Here's how the part is built. I have some questions about the finished solid (model axes, mm). Face numbers are marked on the shaded views. A direction names the side the tool comes from. Give positions to 0.01 mm unless a question says otherwise; leave off trailing zeros. Order: outer loops, then holes, each group sorted by start corner. A loop starts at its lowest first (then second) coordinate and runs counter-clockwise, first axis right, second up. Notation, with made-up numbers: M 69.25,-31.5 L 103.25,-31.5 A12 ccw 103.25,-23.5 Z; hole C -14,45 d4. An arc over 180 degrees is marked long. Use one line per item in the form item = value.
from build123d import *

# Parameters (mm, degrees)
F0_W     = 200
F0_H     = 200
F0_W_2   = 800
F0_H_2   = 800
F1_DEPTH = 200
F2_DEPTH = 300
F3_DEPTH = 200.001
F4_W     = 1200
F4_H     = 1200
F4_W_2   = 800
F4_H_2   = 800
F5_DEPTH = 200


with BuildPart() as f1:
    # F0 (on Top) → F1 (new body)
    with BuildSketch(Plane.XY):
        with Locations((-500, 500)):
            Rectangle(F0_W, F0_H)
        with Locations((0, 500)):
            Rectangle(F0_W_2, F0_H)
        with Locations((500, 500)):
            Rectangle(F0_W, F0_H)
        with Locations((500, 0)):
            Rectangle(F0_W, F0_H_2)
        Rectangle(F0_W_2, F0_H_2)
        with Locations((-500, 0)):
            Rectangle(F0_W, F0_H_2)
        with Locations((-500, -500)):
            Rectangle(F0_W, F0_H)
        with Locations((0, -500)):
            Rectangle(F0_W_2, F0_H)
        with Locations((500, -500)):
            Rectangle(F0_W, F0_H)
    extrude(amount=-F1_DEPTH)

    # F0 (on Top) → F2 (join)
    with BuildSketch(Plane.XY):
        with Locations((-500, -500)):
            Rectangle(F0_W, F0_H)
        with Locations((500, -500)):
            Rectangle(F0_W, F0_H)
        with Locations((500, 500)):
            Rectangle(F0_W, F0_H)
        with Locations((-500, 500)):
            Rectangle(F0_W, F0_H)
    extrude(amount=F2_DEPTH)

    # F0 (on Top) → F3 (cut, through all)
    with BuildSketch(Plane.XY):
        Rectangle(F0_W_2, F0_H_2)
    extrude(amount=-F3_DEPTH, mode=Mode.SUBTRACT)

    # F4 (on face) → F5 (join)
    with BuildSketch(Plane.XY.offset(300)):
        Rectangle(F4_W, F4_H)
        Rectangle(F4_W_2, F4_H_2, mode=Mode.SUBTRACT)
        Polygon((-600, -600), (600, -600), (600, -400), (600, 600), (-600, 600), align=None)
        Rectangle(F4_W_2, F4_H_2, mode=Mode.SUBTRACT)
    extrude(amount=F5_DEPTH)


solid = f1.part
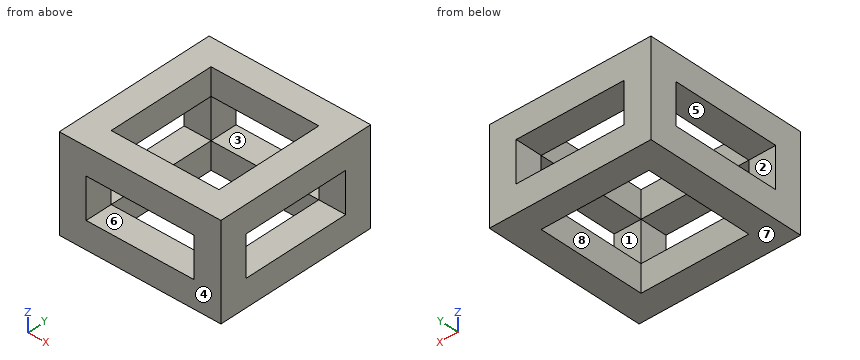
Q1. I want a section at D-D on y = 51. Write out the boundary of the cut face in (x, z), then the cut area to 3 significant figures.
Found:
outline = M -600,-200 L -400,-200 L -400,0 L -600,0 Z; M -600,300 L -400,300 L -400,500 L -600,500 Z; M 400,-200 L 600,-200 L 600,0 L 400,0 Z; M 400,300 L 600,300 L 600,500 L 400,500 Z
area = 160,000 mm²
Q2. I need wall thicknesses on L1, parallel to X at y = 532, z = 168; L2, parallel to Z at x = 427.5, y = -56.5. Which ranges of each line are inside material? Lowest first, please.
Found:
L1 = -600 to -400, 400 to 600
L2 = -200 to 0, 300 to 500
Q3. On a 3-axis mill with a long thin cutter (end or side, diameter ignored), from which of +Z, -Z, +X, -X, +Y, -Y can I reach the whole of each face in a straight line? I mean the marked faces 5, 6, 7 and 8. Say none if no direction works.
Found:
face_5 = +X, -X
face_6 = +Y, -Y
face_7 = -Z, +X, -X, +Y, -Y
face_8 = +Z, -Z
Q4. I want a section at C-C on z = 65. Write out the boundary of the cut face in (x, y), then the cut area to 3 significant figures.
Found:
outline = M -600,-600 L -400,-600 L -400,-400 L -600,-400 Z; M -600,400 L -400,400 L -400,600 L -600,600 Z; M 400,-600 L 600,-600 L 600,-400 L 400,-400 Z; M 400,400 L 600,400 L 600,600 L 400,600 Z
area = 160,000 mm²
Q5. Thinking about a two-plate mould opening in Y: for the marked faces 1, 2, 3 and 4, which applies, +Y half, -Y half, draft (parallel to the pull), parting line (faces both ways), or undercut?
Found:
face_1 = undercut
face_2 = undercut
face_3 = draft
face_4 = -Y half
Q6. I want a section at A-A on y = 425.5. Write out the boundary of the cut face in (x, z).
Found:
outline = M -600,-200 L 600,-200 L 600,500 L -600,500 Z; hole M -400,0 L 400,0 L 400,300 L -400,300 Z
